Model file for the job. Use its own axes, mm. A direction names the side the tool comes from. Round coordinates to 2 decimals unless told otherwise and drop trailing zeros. Loops run counter-clockwise (first coordinate to the right, second up) from the corner with the lowest first, then second, coordinate; pieces in that order, holes last. Notation, with made-up numbers: (80.25, -2) - (130.25, -2) arc R16 cw to (130.25, 3) - close; hole circle Ø4 at (68.25, 40). An arc over 180 degrees is marked (long way). Answer as a JSON object with one key per item and string values.
from build123d import *

# Parameters (mm, degrees)
SKETCH_2_R          = 2.75
EXTRUDE_1_DEPTH     = 6
SKETCH_3_R          = 5
CUT_EXTRUDE_1_DEPTH = 3
FILLET_1_R          = 5
CUT_EXTRUDE_2_DEPTH = 4


with BuildPart() as part:
    # Эскиз2 → Бобышка-Вытянуть1 (new body)
    with BuildSketch(Plane.XY):
        with BuildLine():
            Line((10, 18), (10, -18))
            Line((10, -18), (-10, -18))
            Line((-10, -18), (-10, 18))
            ThreePointArc((-10, 18), (0, 28), (10, 18))
        make_face()
        with Locations((0, 1.5)):
            Circle(SKETCH_2_R, mode=Mode.SUBTRACT)
        with Locations((0, -12.5)):
            Circle(SKETCH_2_R, mode=Mode.SUBTRACT)
        with Locations((0, 18)):
            Circle(SKETCH_2_R, mode=Mode.SUBTRACT)
    extrude(amount=EXTRUDE_1_DEPTH)

    # Эскиз3 → Вырез-Вытянуть1 (cut)
    with BuildSketch(Plane.XY.offset(6)):
        with Locations((0, 1.5)):
            Circle(SKETCH_3_R)
        with Locations((0, -12.5)):
            Circle(SKETCH_3_R)
    extrude(amount=-CUT_EXTRUDE_1_DEPTH, mode=Mode.SUBTRACT)

    # Скругление1
    fillet_1_edges = [part.edges().sort_by_distance(p)[0] for p in [
        (10, -18, 3),
        (-10, -18, 3),
    ]]
    fillet(fillet_1_edges, radius=FILLET_1_R)

    # Эскиз4 → Вырез-Вытянуть2 (cut)
    with BuildSketch(Plane.XY.offset(6)):
        Polygon((2.352702347, 13.925), (4.705404694, 18), (2.352702347, 22.075), (-2.352702347, 22.075), (-4.705404694, 18), (-2.352702347, 13.925), align=None)
    extrude(amount=-CUT_EXTRUDE_2_DEPTH, mode=Mode.SUBTRACT)


solid = part.part
1) Slice it at C-C on x = 0. List the corners of the cut face in (y, z) (3 decimals).
Values follow:
{"outline": "(-18, 0) - (-15.25, 0) - (-15.25, 3) - (-17.5, 3) - (-17.5, 6) - (-18, 6) - close; (-9.75, 0) - (-1.25, 0) - (-1.25, 3) - (-3.5, 3) - (-3.5, 6) - (-7.5, 6) - (-7.5, 3) - (-9.75, 3) - close; (4.25, 0) - (15.25, 0) - (15.25, 2) - (13.925, 2) - (13.925, 6) - (6.5, 6) - (6.5, 3) - (4.25, 3) - close; (20.75, 0) - (28, 0) - (28, 6) - (22.075, 6) - (22.075, 2) - (20.75, 2) - close"}
2) Probe probe 1 along Y at (x, z) = (0, 5.3) (3 decimals); probe 2 along Y at (x, z) = (0, 0.9); probe 3 along X at (y, z) = (1.5, 1.55). List the from-to ranges inside material, lowest first.
Values follow:
{"probe 1": "-18 to -17.5, -7.5 to -3.5, 6.5 to 13.925, 22.075 to 28", "probe 2": "-18 to -15.25, -9.75 to -1.25, 4.25 to 15.25, 20.75 to 28", "probe 3": "-10 to -2.75, 2.75 to 10"}
3) Slice it at A-A on y = 1.5. List the corners of the cut face in (x, z).
Values follow:
{"outline": "(-10, 0) - (-2.75, 0) - (-2.75, 3) - (-5, 3) - (-5, 6) - (-10, 6) - close; (2.75, 0) - (10, 0) - (10, 6) - (5, 6) - (5, 3) - (2.75, 3) - close"}
4) Slice it at D-D on x = -3.5. List the corners of the cut face in (y, z).
Values follow:
{"outline": "(-18, 0) - (27.37, 0) - (27.37, 6) - (20.09, 6) - (20.09, 2) - (15.91, 2) - (15.91, 6) - (5.07, 6) - (5.07, 3) - (-2.07, 3) - (-2.07, 6) - (-8.93, 6) - (-8.93, 3) - (-16.07, 3) - (-16.07, 6) - (-18, 6) - close"}
5) Drop flat-ended pins along their axis: P1, Ø4, axis at x = -1, y = 18.5, coming from the +Z side; P2, Ø3.5, axis at x = 0, y = 18, coming from the -Z side; P3, Ø9, axis at x = 0, y = 1.5, coming from the +Z side. Give the stop position or say it passes through.
Values follow:
{"P1": "z = 2", "P2": "through", "P3": "z = 3"}
6) Two-plate mould, pull along Y, no slides. Class faces 1 (the cylindrical face through (-8, -17, 3)), 2 (the flat face through (2, -15, 3)), 3 (the flat face through (10, 3, 3)): pulls with the +Y half, pulls with the -Y half, needs draft (parallel to the pull), parting line crosses it, or undercut.
Values follow:
{"face 1": "pulls with the -Y half", "face 2": "undercut", "face 3": "needs draft"}
7) Tool access for faces 4 (the cylindrical face through (-0.596, -1.185, 1.479)), 5 (the flat face through (-3.546, 15.991, 4.028)): list every direction of +Z, -Z, +X, -X, +Y, -Y with a clear straight run to the whole face (end or side of a thin tool).
Values follow:
{"face 4": "+Z, -Z", "face 5": "+Z"}
8) Slice it at B-B on z = 5.1. List the corners of the cut face in (x, y) (3 decimals).
Values follow:
{"outline": "(-10, -13) arc R5 ccw to (-5, -18) - (5, -18) arc R5 ccw to (10, -13) - (10, 18) arc R10 ccw to (-10, 18) - close; hole circle Ø10 at (0, -12.5); hole circle Ø10 at (0, 1.5); hole (-4.705, 18) - (-2.353, 13.925) - (2.353, 13.925) - (4.705, 18) - (2.353, 22.075) - (-2.353, 22.075) - close"}
